The listing builds one solid part. Answer for the finished solid, in the listing's coordinates (mm). A direction names the side the tool comes from. Round coordinates to 2 decimals unless told otherwise and drop trailing zeros. Write each loop counter-clockwise with the first axis right and the second up, starting at its lowest first coordinate (ties: lowest second). Pieces come first, ordered by that corner, then holes.
from build123d import *

# Parameters (mm, degrees)
SKETCH1_W           = 762
SKETCH1_H           = 508
SKETCH1_W_2         = 711.2
SKETCH1_H_2         = 457.2
BOSS_EXTRUDE1_DEPTH = 254
SKETCH2_W           = 711.2
SKETCH2_H           = 457.2
BOSS_EXTRUDE2_DEPTH = 25.4
SKETCH3_W           = 76.2
SKETCH3_H           = 76.2
SKETCH3_R           = 6.35
BOSS_EXTRUDE3_DEPTH = 7.62
SKETCH4_R           = 63.5
CUT_EXTRUDE1_DEPTH  = 133.096
SCALE1_SCALE        = 0.5


with BuildPart() as part:
    # Sketch1 → Boss-Extrude1 (new body)
    with BuildSketch(Plane.XY):
        Rectangle(SKETCH1_W, SKETCH1_H)
        Rectangle(SKETCH1_W_2, SKETCH1_H_2, mode=Mode.SUBTRACT)
    extrude(amount=BOSS_EXTRUDE1_DEPTH)

    # Sketch2 → Boss-Extrude2 (add)
    with BuildSketch(Plane.XY.offset(254)):
        Rectangle(SKETCH2_W, SKETCH2_H)
    extrude(amount=-BOSS_EXTRUDE2_DEPTH)

    # Sketch3 → Boss-Extrude3 (add)
    # profile 1 of 4: a face of its own
    with BuildSketch(Plane.XY.offset(254)):
        with Locations((-266.7, -292.1)):
            Rectangle(SKETCH3_W, SKETCH3_H)
        with Locations((-266.7, -292.1)):
            Circle(SKETCH3_R, mode=Mode.SUBTRACT)
    # profile 2 of 4: a face of its own
    with BuildSketch(Plane.XY.offset(254)):
        with Locations((-266.7, 292.1)):
            Rectangle(SKETCH3_W, SKETCH3_H)
        with Locations((-266.7, 292.1)):
            Circle(SKETCH3_R, mode=Mode.SUBTRACT)
    # profile 3 of 4: a face of its own
    with BuildSketch(Plane.XY.offset(254)):
        with Locations((241.3, -292.1)):
            Rectangle(SKETCH3_W, SKETCH3_H)
        with Locations((241.3, -292.1)):
            Circle(SKETCH3_R, mode=Mode.SUBTRACT)
    # profile 4 of 4: a face of its own
    with BuildSketch(Plane.XY.offset(254)):
        with Locations((241.3, 292.1)):
            Rectangle(SKETCH3_W, SKETCH3_H)
        with Locations((241.3, 292.1)):
            Circle(SKETCH3_R, mode=Mode.SUBTRACT)
    extrude(amount=-BOSS_EXTRUDE3_DEPTH)

    # Sketch4 → Cut-Extrude1 (cut)
    with BuildSketch(Plane.XZ.offset(254)):
        with Locations(Location((0, 127, 0), (0, 0, 270))):
            Circle(SKETCH4_R)
    extrude(amount=-CUT_EXTRUDE1_DEPTH, mode=Mode.SUBTRACT)


with BuildPart() as part_1:
    # Scale1: scaled about (0, 0, 0)
    add(part.part.scale(SCALE1_SCALE))


solid = part_1.part
1. For a pull along X with two mould halves and no side action, classify faces 4 (the face through (-190.5, -2, 63)), 5 (the face through (-2, 2, 114.3)), 6 (the face through (125, 146, 123.19)) as released by +X, released by -X, zero draft, split by the parting line, or undercut.
Geometry says:
face 4: released by -X
face 5: undercut
face 6: zero draft
2. A tool of negligible diameter and unlimited length cuts with its end or side. For faces 1 (the face through (-129, -146, 123.19)), 2 (the face through (177.8, -2, 56)), 3 (the face through (1.4, -120.74, 95.22)), from which of +Z, -Z, +X, -X, +Y, -Y can it reach the whole face along a straight path? Write none if from no direction.
Geometry says:
face 1: -Z, +X, -X, -Y
face 2: -Z
face 3: -Y
3. Straight lines are drawn through the part: line 1 along Y through (x, z) = (-133.35, 124) (3 decimals); line 2 along X through (y, z) = (-146, 124); line 3 along X through (y, z) = (-117, 63). For each, find the intervals that lie inside material, in ascending order.
Geometry says:
line 1: y = -165.1 to -149.225, -142.875 to 142.875, 149.225 to 165.1
line 2: x = -152.4 to -136.52, -130.18 to -114.3, 101.6 to 117.48, 123.82 to 139.7
line 3: x = -190.5 to -31.75, 31.75 to 190.5
4. Given pin 1 (1.9 mm diameter, centred on y = 138, z = 124.5, fed in from -X); pin 2 (12 mm diameter, centred on x = -32.5, z = 76.5, fed in from -Y); pin 3 (11.5 mm diameter, centred on x = 130, y = -144.5, fed in from -Z), each flat-ended and moving along its own axis, determine where each tip first touches the part or whether it passes through.
Geometry says:
pin 1: stops at x = -152.4
pin 2: stops at y = -127
pin 3: stops at z = 123.19
5. Section B-B on z = 25 is taken. Determine the outline of the cut face in (x, y), plus the area to 3 significant figures.
Geometry says:
outline: (-190.5, -127) - (190.5, -127) - (190.5, 127) - (-190.5, 127) - close; hole (-177.8, -114.3) - (177.8, -114.3) - (177.8, 114.3) - (-177.8, 114.3) - close
area: 15,500 mm2
6. Section C-C on x = 134 is taken. Determine the outline of the cut face in (y, z), plus the area to 3 significant figures.
Geometry says:
outline: (-165.1, 123.19) - (-127, 123.19) - (-127, 0) - (-114.3, 0) - (-114.3, 114.3) - (114.3, 114.3) - (114.3, 0) - (127, 0) - (127, 123.19) - (165.1, 123.19) - (165.1, 127) - (-165.1, 127) - close
area: 6,420 mm2
7. Section A-A on x = 0 is taken. Determine the outline of the cut face in (y, z).
Geometry says:
outline: (-127, 0) - (-114.3, 0) - (-114.3, 31.75) - (-127, 31.75) - close; (-127, 95.25) - (-114.3, 95.25) - (-114.3, 114.3) - (114.3, 114.3) - (114.3, 0) - (127, 0) - (127, 127) - (-127, 127) - close
8. Section D-D on y = 12.5 is taken. Determine the outline of the cut face in (x, z).
Geometry says:
outline: (-190.5, 0) - (-177.8, 0) - (-177.8, 114.3) - (177.8, 114.3) - (177.8, 0) - (190.5, 0) - (190.5, 127) - (-190.5, 127) - close
